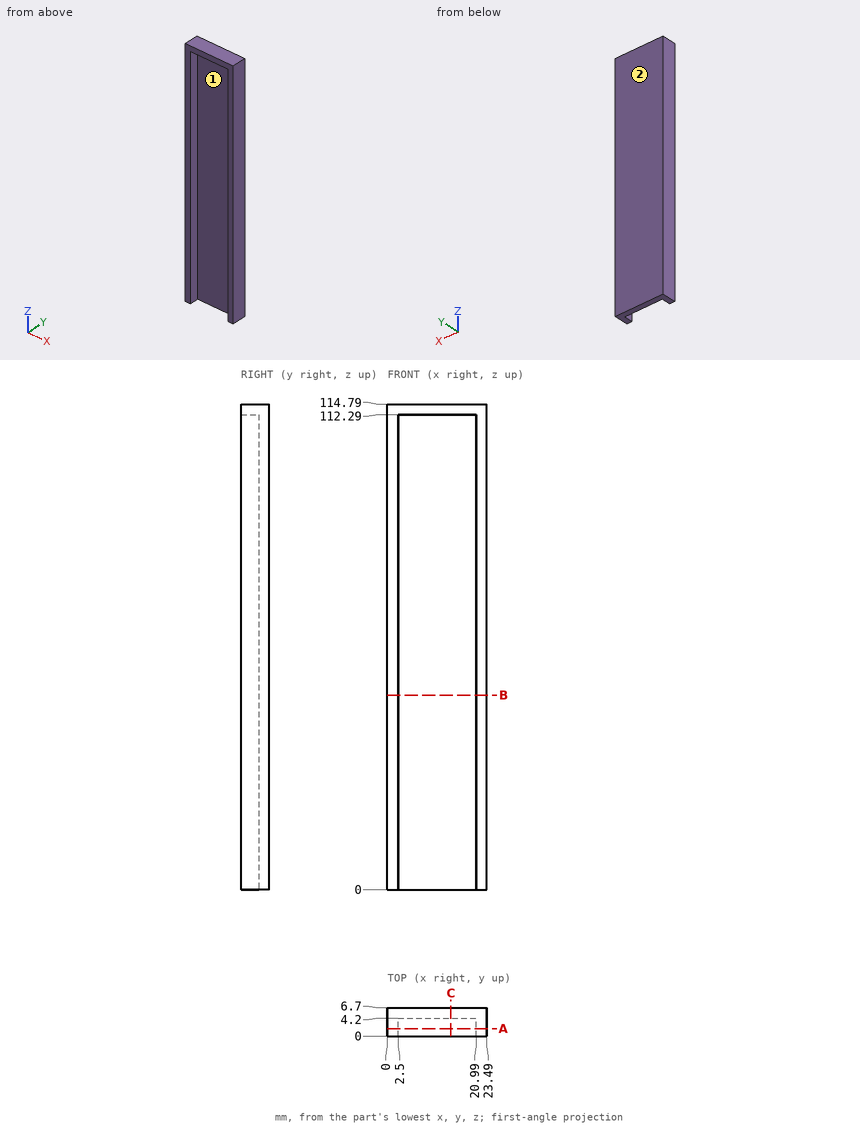
Geometry: see drawing. Coordinates: mm, zero at the bounding-box minimum. Coordinates: 2 decimals unless noted, no trailing zeros. Order: outer loops, then holes, each group sorted by start corner. A loop starts at its lowest first (then second) coordinate and runs counter-clockwise, first axis right, second up. Notation, with made-up numbers: (66, 68.5) - (118, 68.5) arc R19 ccw to (118, 86.5) - close; hole circle Ø11 at (74.25, -35.75). An arc over 180 degrees is marked (long way). Return JSON: item names as keys, results as strings.
Q1. Cut plane B-B (z = 46). Return loops of the section in (x, y).
The answers:
{"outline": "(0, 0) - (2.5, 0) - (2.5, 4.2) - (20.99, 4.2) - (20.99, 0) - (23.49, 0) - (23.49, 6.7) - (0, 6.7) - close"}
Q2. First-contact query: pin 1 (1.5 mm diameter, centred on x = 13, z = 17.5, fed in from -Y). Flat tip, straight axial feed; report the tip coordinate or a pass-through.
The answers:
{"pin 1": "stops at y = 4.2"}
Q3. Draft query along X for the marked faces 1 and 2. Return one class per face: +X half, -X half, draft (parallel to the pull), parting line (faces both ways), or undercut.
The answers:
{"face 1": "undercut", "face 2": "draft"}
Q4. Cut plane C-C (x = 15). Return loops of the section in (y, z).
The answers:
{"outline": "(0, 112.29) - (4.2, 112.29) - (4.2, 0) - (6.7, 0) - (6.7, 114.79) - (0, 114.79) - close"}
Q5. Ray query, probe 1 along X at (y, z) = (1, 51); probe 2 along Y at (x, z) = (8.75, 58); probe 3 along Z at (x, y) = (2.75, 0.5). Return the intervals inside material, ascending.
The answers:
{"probe 1": "x = 0 to 2.5, 20.99 to 23.49", "probe 2": "y = 4.2 to 6.7", "probe 3": "z = 112.29 to 114.79"}
Q6. Cut plane A-A (y = 1.75). Return loops of the section in (x, z).
The answers:
{"outline": "(0, 0) - (2.5, 0) - (2.5, 112.29) - (20.99, 112.29) - (20.99, 0) - (23.49, 0) - (23.49, 114.79) - (0, 114.79) - close"}
